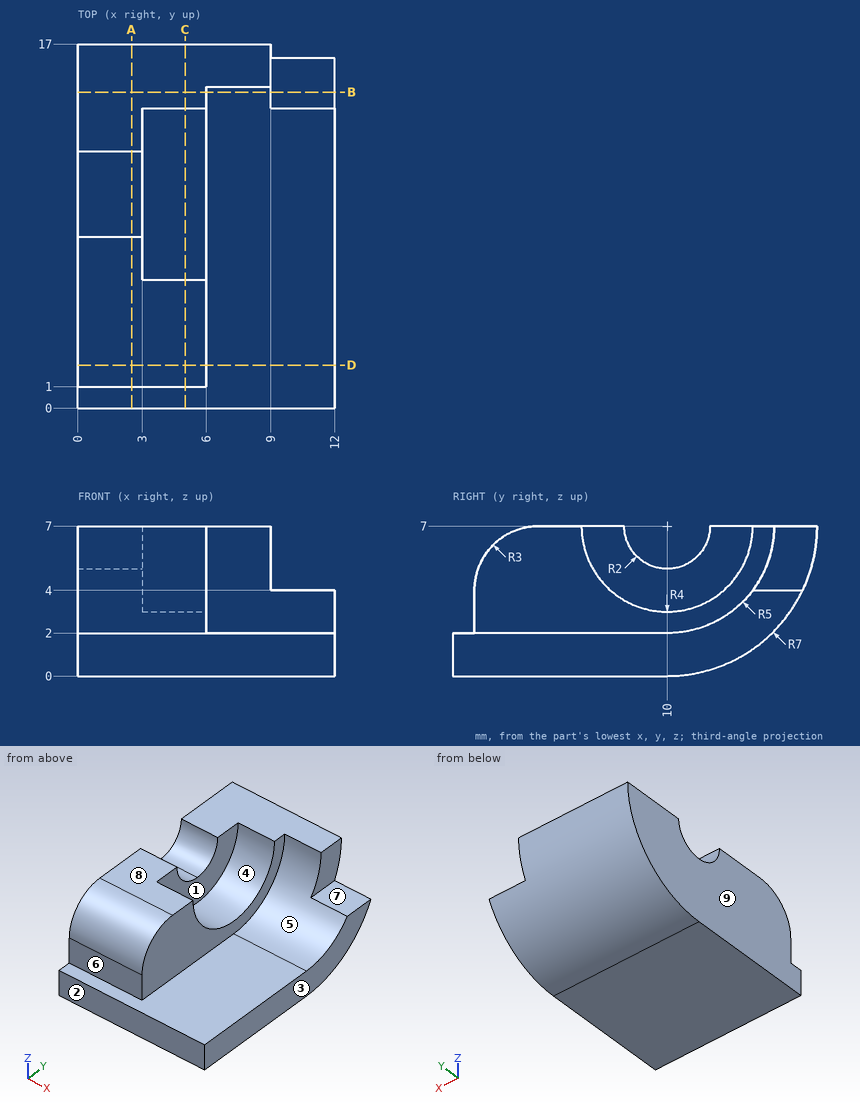
Could you check a few things on this drawing? It's one solid part, dimensions in mm from its lowest x, y, z. A direction names the side the tool comes from. Coordinates: 2 decimals unless noted, no trailing zeros. Order: outer loops, then holes, each group sorted by start corner. A loop starts at its lowest first (then second) coordinate and runs counter-clockwise, first axis right, second up. Notation, with made-up numbers: M 14,84.25 L 63,84.25 A12 ccw 63,94.25 Z; hole C 27,-2.75 d6. An arc over 180 degrees is marked long. Answer as a JSON object with one key per item and string values. Group by question number.
(1) For pin 1 (0.9 mm diameter, centred on y = 16, z = 6, fed in from +X); pin 2 (0.6 mm diameter, centred on x = 3.5, z = 3, fed in from -Y); pin 3 (3 mm diameter, centred on y = 11.5, z = 4.5, fed in from +X), each with a flat end and sliding along its axis, tell me the tip position at first contact or that it passes through.
(2) Suppose I cut it at D-D, the plane y = 2. Please give me the cut outline in (x, z).
(3) Suppose I cut it at A-A, the plane x = 2.5. Please give me the cut outline in (y, z).
(4) Suppose I cut it at C-C, the plane x = 5. Please give me the cut outline in (y, z), then the cut area to 3 significant figures.
(5) If we mould it in two halves opening along Y, with no side actions, what happens to the marked faces 1, 2, 3 and 4? For each: released by +Y, released by -Y, zero draft, split by the parting line, or undercut.
(6) Which directions (+Z, -Z, +X, -X, +Y, -Y) give clear straight access to the entire face, cutting with the end or side of a thin tool? Please do the marked faces 5, 6, 7, 8 and 9.
(7) Suppose I cut it at B-B, the plane y = 14.75. Please give me the cut outline in (x, z), then the cut area to 3 significant figures.
(8) I need wall thicknesses on probe 1 along X at (y, z) = (3, 6); probe 2 along Z at (x, y) = (8, 7.25); probe 3 along Y at (x, z) = (7, 4). Which ranges of each line are inside material? Lowest first, please.
Values found:
{
 "1": {"pin 1": "stops at x = 9", "pin 2": "stops at y = 1", "pin 3": "stops at x = 6"},
 "2": {"outline": "M 0,0 L 12,0 L 12,2 L 6,2 L 6,6.24 L 0,6.24 Z"},
 "3": {"outline": "M 0,0 L 10,0 A7 ccw 17,7 L 12,7 A2 cw 8,7 L 4,7 A3 ccw 1,4 L 1,2 L 0,2 Z"},
 "4": {"outline": "M 0,0 L 10,0 A7 ccw 17,7 L 14,7 A4 cw 6,7 L 4,7 A3 ccw 1,4 L 1,2 L 0,2 Z", "area": "76.4 mm^2"},
 "5": {"face 1": "undercut", "face 2": "released by -Y", "face 3": "zero draft", "face 4": "undercut"},
 "6": {"face 5": "+Z, +X, -Y", "face 6": "+Z, +X, -X, -Y", "face 7": "+Z, +X, +Y, -Y", "face 8": "+Z, +X, -X, +Y, -Y", "face 9": "+Z, -Z, -X, +Y, -Y"},
 "7": {"outline": "M 0,1.86 L 12,1.86 L 12,4 L 9,4 L 9,5.44 L 6,5.44 L 6,7 L 0,7 Z", "area": "48.0 mm^2"},
 "8": {"probe 1": "x = 0 to 6", "probe 2": "z = 0 to 2", "probe 3": "y = 14 to 16.32"}
}
